Build history of the part. All positions in model axes, mm. Face numbers are marked on the shaded views. A direction names the side the tool comes from. Give positions to 0.01 mm unless a question says otherwise; leave off trailing zeros. Write each loop counter-clockwise with the first axis right and the second up, starting at its lowest first coordinate (ties: lowest second). Pieces come first, ordered by that corner, then holes.
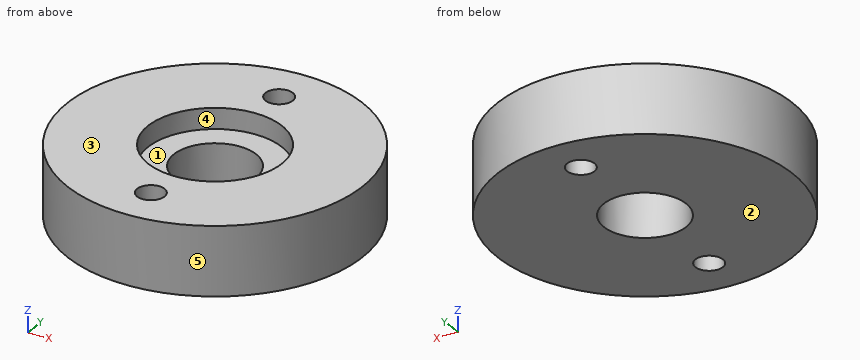
from build123d import *

# Parameters (mm, degrees)
CYLINDER010_R               = 2
CYLINDER010_DEPTH           = 15
CYLINDER011_R               = 2
CYLINDER011_DEPTH           = 15
CYLINDER011_PLACEMENT_ANGLE = 1
CYLINDER009_R               = 6
CYLINDER009_DEPTH           = 20
CYLINDER007_R               = 9.75
CYLINDER007_DEPTH           = 6
CYLINDER003_R               = 21.5
CYLINDER003_DEPTH           = 10
CUT005_PLACEMENT_ANGLE      = 180


with BuildPart() as cylinder010:
    # Cylinder010 → Cylinder010 (new body)
    with BuildSketch(Plane(origin=(0, 15, -1), x_dir=(1, 0, 0), z_dir=(0, 0, 1))):
        Circle(CYLINDER010_R)
    extrude(amount=CYLINDER010_DEPTH)


with BuildPart() as fusion003:
    # Cylinder011 → Cylinder011 (new body)
    with BuildSketch(Plane.XY):
        Circle(CYLINDER011_R)
    extrude(amount=CYLINDER011_DEPTH)


with BuildPart() as fusion003_1:
    # Cylinder011 placement: moved
    add(fusion003.part.moved(Location((0, -15, -1))).rotate(Axis((0, -15, -1), (0, 0, 1)), CYLINDER011_PLACEMENT_ANGLE))

    # Fusion003: union Cylinder010
    add(cylinder010.part)


with BuildPart() as cylinder009:
    # Cylinder009 → Cylinder009 (new body)
    with BuildSketch(Plane.XY):
        Circle(CYLINDER009_R)
    extrude(amount=CYLINDER009_DEPTH)


with BuildPart() as cylinder007:
    # Cylinder007 → Cylinder007 (new body)
    with BuildSketch(Plane.XY):
        Circle(CYLINDER007_R)
    extrude(amount=CYLINDER007_DEPTH)


with BuildPart() as small_bearing_ring001:
    # Cylinder003 → Cylinder003 (new body)
    with BuildSketch(Plane.XY.offset(3)):
        Circle(CYLINDER003_R)
    extrude(amount=CYLINDER003_DEPTH)

    # Cut006: cut Cylinder007
    add(cylinder007.part, mode=Mode.SUBTRACT)

    # Cut005: cut Cylinder009
    add(cylinder009.part, mode=Mode.SUBTRACT)


with BuildPart() as small_bearing_ring001_1:
    # Cut005 placement: moved
    add(small_bearing_ring001.part.moved(Location((0, 0, 13))).rotate(Axis((0, 0, 13), (0, 1, 0)), CUT005_PLACEMENT_ANGLE))

    # Cut008: cut Fusion003
    add(fusion003_1.part, mode=Mode.SUBTRACT)


with BuildPart() as small_bearing_ring001_2:
    # Cut008 placement: moved
    add(small_bearing_ring001_1.part.moved(Location((0, -57, 0))))


solid = small_bearing_ring001_2.part
1. Saw through at D-D on y = -42. Give the cut face in (x, z).
2. Saw through at A-A on y = -57. Give the cut face in (x, z).
3. Mould opens along Y. For the marked faces 3, 4 and 5 say: pulls with the +Y half, pulls with the -Y half, needs draft (parallel to the pull), parting line crosses it, or undercut.
4. 3-axis set-ups, long thin cutter, end or side, ignore diameter. For the marked faces 1 and 2: which of +Z, -Z, +X, -X, +Y, -Y reach the whole face in a straight line?
5. Drop flat-ended pins along their axis: pin 1 (2 mm diameter, centred on x = -0.5, z = 1.5, fed in from +Y); pin 2 (6 mm diameter, centred on y = -53, z = 3.5, fed in from -X); pin 3 (6 mm diameter, centred on x = 14, z = 5.5, fed in from -Y); pin 4 (3 mm diameter, centred on x = 0, y = -72, fed in from -Z) (1 decimal). Give the stop position or say it passes through.
6. Drill centre lines: line 1 along Y through (x, z) = (0, 6); line 2 along X through (y, z) = (-41, 4.25); line 3 along Y through (x, z) = (-0.5, 6.5). Where is each one in solid material? Low to high.
7. Saw through at B-B on x = 0. Give the cut face in (y, z), plus the area to 4 significant figures.
8. Saw through at C-C on x = 5.5. Give the cut face in (y, z), plus the area to 3 significant figures.
Outcome:
1. outline: (-15.4, 0) - (-2, 0) - (-2, 10) - (-15.4, 10) - close; (2, 0) - (15.4, 0) - (15.4, 10) - (2, 10) - close
2. outline: (-21.5, 0) - (-6, 0) - (-6, 7) - (-9.75, 7) - (-9.75, 10) - (-21.5, 10) - close; (6, 0) - (21.5, 0) - (21.5, 10) - (9.75, 10) - (9.75, 7) - (6, 7) - close
3. face 3: needs draft
3. face 4: undercut
3. face 5: parting line crosses it
4. face 1: +Z
4. face 2: -Z, +X, -X, +Y, -Y
5. pin 1: stops at y = -35.5
5. pin 2: stops at x = -21.48
5. pin 3: stops at y = -75.47
5. pin 4: passes through
6. line 1: y = -78.5 to -74, -70 to -63, -51 to -44, -40 to -35.5
6. line 2: x = -14.36 to -1.73, 1.73 to 14.36
6. line 3: y = -78.49 to -73.94, -70.06 to -62.98, -51.02 to -43.94, -40.06 to -35.51
7. outline: (-78.5, 0) - (-74, 0) - (-74, 10) - (-78.5, 10) - close; (-70, 0) - (-63, 0) - (-63, 7) - (-66.75, 7) - (-66.75, 10) - (-70, 10) - close; (-51, 0) - (-44, 0) - (-44, 10) - (-47.25, 10) - (-47.25, 7) - (-51, 7) - close; (-40, 0) - (-35.5, 0) - (-35.5, 10) - (-40, 10) - close
7. area: 207.5 mm2
8. outline: (-77.78, 0) - (-59.4, 0) - (-59.4, 7) - (-65.05, 7) - (-65.05, 10) - (-77.78, 10) - close; (-54.6, 0) - (-36.22, 0) - (-36.22, 10) - (-48.95, 10) - (-48.95, 7) - (-54.6, 7) - close
8. area: 334 mm2
